Check sheet for the modelled part. Datum: model origin and axes. Units: mm. A direction names the side the tool comes from. Give positions to 0.01 mm unless a question says otherwise; leave off trailing zeros. Loops run counter-clockwise (first coordinate to the right, second up) from the corner with the lowest first, then second, coordinate; pieces in that order, holes last. Notation, with made-up numbers: (59.25, 29.5) -> (115.25, 29.5) arc R31 cw to (115.25, 61.5) -> close; hole circle Ø3 at (58, 22.5). An arc over 180 degrees is marked (long way). Write each question's results on one line, items separated by ' | '. Start each with the question number.
Item 1: Cross-section at A-A on x = -52. Enter the section's corners in (y, z), then the cut area to 3 significant figures.
Item 2: Cross-section at B-B on x = 19. Enter the section's corners in (y, z).
Item 3: Scan lines: line 1 along X through (y, z) = (11.5, 5); line 2 along Y through (x, z) = (-40, 3); line 3 along Y through (x, z) = (66.5, 2). Record each from-to range of solid material in increasing order.
Item 4: Mould release check, pull along Y, two halves, no side actions. Record for faces 1 (the face through (-0.58, 26.31, 3.57)), 2 (the face through (22, 44, 3)), 3 (the face through (23, 36, 3)), 4 (the face through (73, -74, 3)): pulls with the +Y half, pulls with the -Y half, needs draft (parallel to the pull), parting line crosses it, or undercut.
Item 5: Cross-section at C-C on y = 26. Enter the section's corners in (x, z).
Item 6: Gauge pin test, flat ends, axial feed: pin 1 Ø1.8 at (x, z) = (-6, 4.5) entering from +Y (3 decimals); pin 2 Ø2 at (x, z) = (62.5, 4.5) entering from -Y; pin 3 Ø1.4 at (x, z) = (73, 5) entering from +Y. Record the tip position at first contact, or that the pin passes through.
Item 7: Access from +Z, -Z, +X, -X, +Y, -Y to the whole of each face (thin tool, end or side, straight path). Record for faces 5 (the face through (-50, -22.5, 3)), 6 (the face through (-50, 21.3, 4)), 7 (the face through (-50, 22.5, 3)), 8 (the face through (24.44, -39.89, 2.96)).
from build123d import *

# Parameters (mm, degrees)
PAD_DEPTH   = 6
THICKNESS_T = -1.2


with BuildPart() as part:
    # Sketch → Pad (new body)
    with BuildSketch(Plane.XY):
        Polygon((80, -74), (65, -74), (-15, -22.5), (-85, -22.5), (-85, 22.5), (-15, 22.5), (15, 44), (30, 44), (30, 36), (15, 36), (-15, 14.5), (-15, 4), (0, 4), (0, -4), (-15, -4), (-15, -14.5), (65, -66), (80, -66), align=None)
    extrude(amount=PAD_DEPTH)

    # Thickness
    thickness_openings = [part.faces().sort_by_distance(p)[0] for p in [
        (-29.840547, -5.671982, 6),
    ]]
    offset(amount=THICKNESS_T, openings=thickness_openings, kind=Kind.INTERSECTION)


solid = part.part
Answer sheet:
1) outline: (-22.5, 0) -> (22.5, 0) -> (22.5, 6) -> (21.3, 6) -> (21.3, 1.2) -> (-21.3, 1.2) -> (-21.3, 6) -> (-22.5, 6) -> close | area: 65.5 mm²
2) outline: (-44.39, 0) -> (-36.39, 0) -> (-36.39, 6) -> (-37.81, 6) -> (-37.81, 1.2) -> (-42.96, 1.2) -> (-42.96, 6) -> (-44.39, 6) -> close; (36, 0) -> (44, 0) -> (44, 6) -> (42.8, 6) -> (42.8, 1.2) -> (37.2, 1.2) -> (37.2, 6) -> (36, 6) -> close
3) line 1: x = -85 to -83.8, -16.2 to -15 | line 2: y = -22.5 to -21.3, 21.3 to 22.5 | line 3: y = -74 to -72.8, -67.2 to -66
4) face 1: undercut | face 2: pulls with the +Y half | face 3: undercut | face 4: pulls with the -Y half
5) outline: (-10.12, 0) -> (1.05, 0) -> (1.05, 6) -> (-1.01, 6) -> (-1.01, 1.2) -> (-8.06, 1.2) -> (-8.06, 6) -> (-10.12, 6) -> close
6) pin 1: stops at y = 29.595 | pin 2: stops at y = -73.03 | pin 3: stops at y = -66
7) face 5: +Z, -Z, -X, -Y | face 6: +Z | face 7: +Z, -Z, -X, +Y | face 8: +Z, -Z, +X
